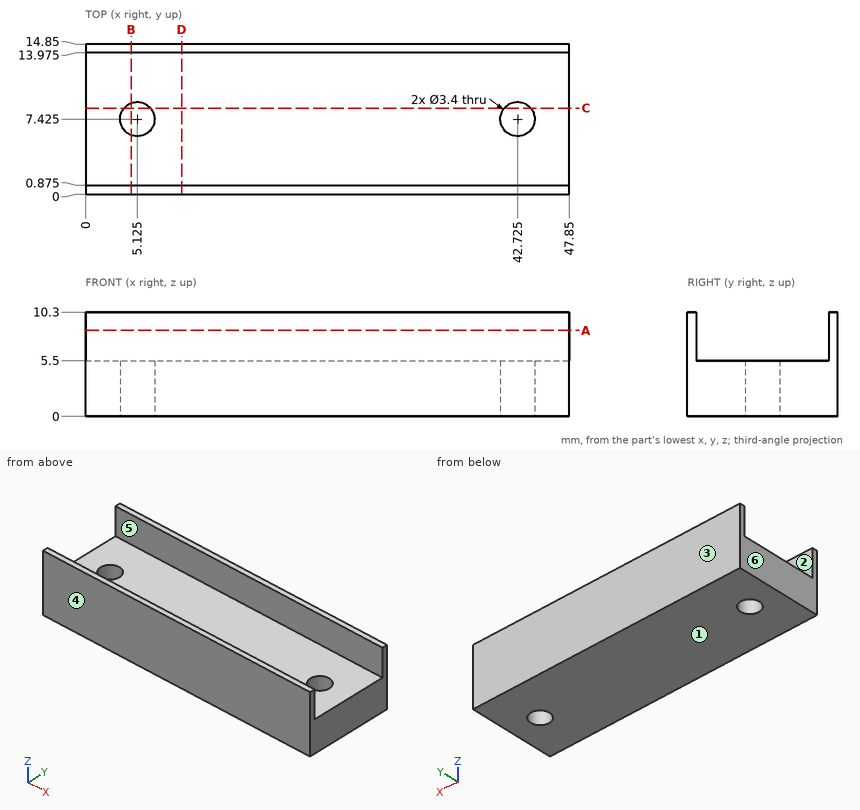
Drawing for the job (mm, zero at the part's lowest x, y, z). A direction names the side the tool comes from. Coordinates: 2 decimals unless noted, no trailing zeros. Write each loop counter-clockwise with the first axis right and the second up, starting at its lowest first coordinate (ties: lowest second). Pieces come first, ordered by that corner, then holes. Notation, with made-up numbers: (13, -10) -> (55, -10) arc R27 ccw to (55, 8) -> close; hole circle Ø2 at (38, 45). An arc over 180 degrees is marked (long way). One line per item, written item: value. Start each with the question number.
1) Flat gauge pins, fed straight in: pin 1 Ø4 at (x, z) = (29, 8) entering from -Y; pin 2 Ø6.5 at (x, y) = (30, 6) entering from +Z. Where does each tip first touch, or does it go through?
2) Pull direction Y, two halves, no side cores. Call the marked faces 3, 4, 5 and 6: +Y half, -Y half, draft (parallel to the pull), parting line (faces both ways), or undercut.
3) Slice it at C-C on y = 8.5. Write the cut outline in (x, z).
4) Slice it at D-D on x = 9.5. Write the cut outline in (y, z) (3 decimals).
5) Slice it at B-B on x = 4.5. Write the cut outline in (y, z) (3 decimals).
6) Slice it at A-A on z = 8.5. Write the cut outline in (x, y) (3 decimals).
7) Which spindle directions (+Z, -Z, +X, -X, +Y, -Y) get a long thin tool onto all of the face, cutting with end or side? Do the marked faces 1 and 2. Say none if no direction does.
8) Probe probe 1 along Y at (x, z) = (40.5, 7) (3 decimals); probe 2 along Z at (x, y) = (45, 6.5); probe 3 along Y at (x, z) = (6, 5). List the from-to ranges inside material, lowest first.
Answers follow:
1. pin 1: y = 0
1. pin 2: z = 5.5
2. face 3: +Y half
2. face 4: -Y half
2. face 5: undercut
2. face 6: draft
3. outline: (0, 0) -> (3.81, 0) -> (3.81, 5.5) -> (0, 5.5) -> close; (6.44, 0) -> (41.41, 0) -> (41.41, 5.5) -> (6.44, 5.5) -> close; (44.04, 0) -> (47.85, 0) -> (47.85, 5.5) -> (44.04, 5.5) -> close
4. outline: (0, 0) -> (14.85, 0) -> (14.85, 10.3) -> (13.975, 10.3) -> (13.975, 5.5) -> (0.875, 5.5) -> (0.875, 10.3) -> (0, 10.3) -> close
5. outline: (0, 0) -> (5.844, 0) -> (5.844, 5.5) -> (0.875, 5.5) -> (0.875, 10.3) -> (0, 10.3) -> close; (9.006, 0) -> (14.85, 0) -> (14.85, 10.3) -> (13.975, 10.3) -> (13.975, 5.5) -> (9.006, 5.5) -> close
6. outline: (0, 0) -> (47.85, 0) -> (47.85, 0.875) -> (0, 0.875) -> close; (0, 13.975) -> (47.85, 13.975) -> (47.85, 14.85) -> (0, 14.85) -> close
7. face 1: -Z, +X, -X, +Y, -Y
7. face 2: +Z, +X, -X
8. probe 1: 0 to 0.875, 13.975 to 14.85
8. probe 2: 0 to 5.5
8. probe 3: 0 to 5.97, 8.88 to 14.85
